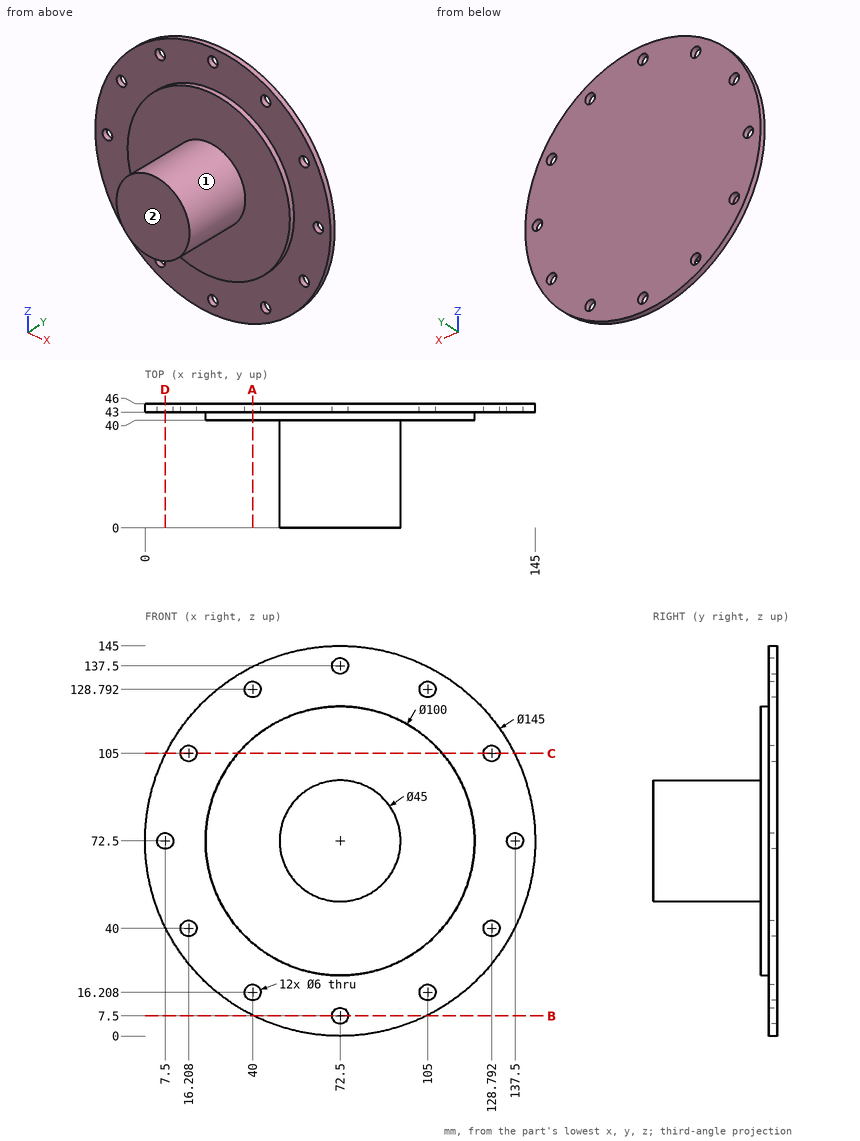
Answer from the drawing. Dimensions are ordinates in mm from the lowest x, y and z of the part. A direction names the side the tool comes from. Round coordinates to 2 decimals unless told otherwise and drop trailing zeros. Write each loop counter-clockwise with the first axis right and the second up, starting at its lowest first coordinate (ties: lowest second). Pieces come first, ordered by that corner, then holes. Notation, with made-up numbers: (-20, -24) -> (3, -24) arc R9 ccw to (3, -11) -> close; hole circle Ø9 at (78.5, 51). An arc over 180 degrees is marked (long way). Answer in a Markdown table with one row per item. Add a question column.
1) Which of the six approach directions +Z, -Z, +X, -X, +Y, -Y give full straight-line access (tool end or side, diameter ignored) to the marked faces 1 and 2?
2) Find section D-D, the plane x = 7.5. Determine the outline of the cut face in (y, z).
3) Find section C-C, the plane z = 105. Determine the outline of the cut face in (x, y), and give its area (3 significant figures).
4) Find section B-B, the plane z = 7.5. Determine the outline of the cut face in (x, y).
5) Consider line 1 (X direction, y = 45.2, z = 105); line 2 (Y direction, x = 105, z = 58.5); line 3 (Y direction, x = 31, z = 19). Determine where each line is inside the solid, lowest interval first.
6) Find section A-A, the plane x = 40. Determine the outline of the cut face in (y, z).
7) Given P1, Ø9.5, axis at x = 72.5, z = 7.5, coming from the -Y side; P2, Ø5, axis at x = 40, z = 128.79, coming from the -Y side; P3, Ø9.5, axis at x = 40, z = 16.21, coming from the +Y side, each flat-ended and moving along its own axis, determine where each tip first touches the part or whether it passes through.
Findings below:
| question | item | result |
|---|---|---|
| 1 | face 1 | -Y |
| 1 | face 2 | +Z, -Z, +X, -X, -Y |
| 2 | outline | (43, 40.39) -> (46, 40.39) -> (46, 69.5) -> (43, 69.5) -> close; (43, 75.5) -> (46, 75.5) -> (46, 104.61) -> (43, 104.61) -> close |
| 3 | outline | (7.69, 43) -> (13.21, 43) -> (13.21, 46) -> (7.69, 46) -> close; (19.21, 43) -> (34.5, 43) -> (34.5, 40) -> (110.5, 40) -> (110.5, 43) -> (125.79, 43) -> (125.79, 46) -> (19.21, 46) -> close; (131.79, 43) -> (137.31, 43) -> (137.31, 46) -> (131.79, 46) -> close |
| 3 | area | 581 mm² |
| 4 | outline | (40.39, 43) -> (69.5, 43) -> (69.5, 46) -> (40.39, 46) -> close; (75.5, 43) -> (104.61, 43) -> (104.61, 46) -> (75.5, 46) -> close |
| 5 | line 1 | 7.69 to 13.21, 19.21 to 125.79, 131.79 to 137.31 |
| 5 | line 2 | 40 to 46 |
| 5 | line 3 | 43 to 46 |
| 6 | outline | (40, 34.5) -> (43, 34.5) -> (43, 19.21) -> (46, 19.21) -> (46, 125.79) -> (43, 125.79) -> (43, 110.5) -> (40, 110.5) -> close; (43, 7.69) -> (46, 7.69) -> (46, 13.21) -> (43, 13.21) -> close; (43, 131.79) -> (46, 131.79) -> (46, 137.31) -> (43, 137.31) -> close |
| 7 | P1 | y = 43 |
| 7 | P2 | through |
| 7 | P3 | y = 46 |
